from build123d import *

# Parameters (mm, degrees)
BOSS_EXTRUDE7_DEPTH = 40
BOSS_EXTRUDE8_DEPTH = 10
SKETCH16_R          = 4
CUT_EXTRUDE6_DEPTH  = 93.663838512
SKETCH17_R          = 4.375
CUT_EXTRUDE7_DEPTH  = 10
FILLET2_R           = 5
MIRROR2_START       = 14.3750001
MIRROR2_DEPTH       = 6.6249998
MIRROR2_2_DEPTH     = 10
MIRROR2_START_2     = 5
MIRROR2_3_DEPTH     = 0.6249999
MIRROR2_START_3     = 34.3750001
MIRROR2_4_DEPTH     = 0.6249999
MIRROR2_5_DEPTH     = 40
MIRROR2_START_4     = -9.5
MIRROR2_6_OUTLINE_R = 4.375
MIRROR2_6_DEPTH     = 8
MIRROR2_START_5     = 18.089296501
MIRROR2_7_OUTLINE_R = 4
MIRROR2_7_DEPTH     = 10.910703499


with BuildPart() as part:
    # Sketch15 → Boss-Extrude7 (new body)
    with BuildSketch(Plane(origin=(0, 0, 0), x_dir=(0, 0, -1), z_dir=(0, 1, 0))):
        with BuildLine():
            Line((33, 0), (39.3, 0))
            Line((39.3, 0), (69, -29.7))
            Line((69, -29.7), (55.282128445, -29.7))
            Line((55.282128445, -29.7), (40.368228689, -14.786100244))
            Line((40.368228689, -14.786100244), (27.577164466, -27.577164466))
            ThreePointArc((27.577164466, -27.577164466), (-10.389986255, -37.590533191), (-37.825256113, -9.5))
            Line((-37.825256113, -9.5), (-52.815891464, -9.5))
            Line((-52.815891464, -9.5), (-52.815891464, -1.5))
            Line((-52.815891464, -1.5), (-32.965891464, -1.5))
            ThreePointArc((-32.965891464, -1.5), (0.750193874, -32.991471764), (33, 0))
        make_face()
    extrude(amount=BOSS_EXTRUDE7_DEPTH)

    # Sketch15_4 → Boss-Extrude8 (add)
    with BuildSketch(Plane(origin=(0, 0, 0), x_dir=(0, 0, -1), z_dir=(0, 1, 0))):
        with BuildLine():
            ThreePointArc((27.577164466, -27.577164466), (26.44822372, -28.661672353), (25.276669084, -29.7))
            Line((25.276669084, -29.7), (55.282128445, -29.7))
            Line((55.282128445, -29.7), (40.368228689, -14.786100244))
            Line((40.368228689, -14.786100244), (27.577164466, -27.577164466))
        make_face()
    extrude(amount=BOSS_EXTRUDE8_DEPTH)

    # Sketch16 → Cut-Extrude6 (cut, through all)
    with BuildSketch(Plane(origin=(-12.791064222, 0, -12.791064222), x_dir=(-0.707106781186546, 0, 0.707106781186549), z_dir=(0.707106781186549, 0, 0.707106781186546))):
        with Locations(Location((-53.189296501, -25, 0), (0, 0, 180))):
            Circle(SKETCH16_R)
    extrude(amount=-CUT_EXTRUDE6_DEPTH, mode=Mode.SUBTRACT)

    # Sketch17 → Cut-Extrude7 (cut)
    with BuildSketch(Plane(origin=(0, 0, 0), x_dir=(0, -1, 0), z_dir=(1, 0, 0))):
        with Locations(Location((-30, -45.320573788, 0), (0, 0, 270))):
            Circle(SKETCH17_R)
        with Locations(Location((-10, -45.320573788, 0), (0, 0, 270))):
            Circle(SKETCH17_R)
    extrude(amount=CUT_EXTRUDE7_DEPTH, mode=Mode.SUBTRACT)

    # Fillet2
    fillet2_edges = [part.edges().sort_by_distance(p)[0] for p in [
        (5.5, 0, 52.815891464),
        (5.5, 40, 52.815891464),
        (14.786100244, 25, -40.368228689),
    ]]
    fillet(fillet2_edges, radius=FILLET2_R)

    # Mirror2: read off the stored shape, not the designer's step
    # Mirror2 outline → Mirror2 (add)
    with BuildSketch(Plane(origin=(0, 0, 0), x_dir=(1, 0, 0), z_dir=(0, 1, 0)).offset(MIRROR2_START)):
        with BuildLine():
            ThreePointArc((-27.577164466, 27.577164466), (-37.590533191, -10.389986255), (-9.5, -37.825256113))
            Line((-9.5, -37.825256113), (-9.5, -52.815891464))
            Line((-9.5, -52.815891464), (-1.5, -52.815891464))
            Line((-1.5, -52.815891464), (-1.5, -32.965891464))
            ThreePointArc((-1.5, -32.965891464), (-32.991471764, 0.750193874), (0, 33))
            Line((0, 33), (0, 39.3))
            Line((0, 39.3), (-29.7, 69))
            Line((-29.7, 69), (-29.7, 55.282128445))
            Line((-29.7, 55.282128445), (-18.32163415, 43.903762595))
            ThreePointArc((-18.32163415, 43.903762595), (-16.857168056, 40.368228689), (-18.32163415, 36.832694783))
            Line((-18.32163415, 36.832694783), (-27.577164466, 27.577164466))
        make_face()
    extrude(amount=MIRROR2_DEPTH)



with BuildPart() as body_2:
    # Mirror2 2 outline → Mirror2 2 (new body)
    with BuildSketch(Plane(origin=(0, 0, 0), x_dir=(1, 0, 0), z_dir=(0, 1, 0))):
        with BuildLine():
            Line((-29.7, 55.282128445), (-29.7, 25.276669084))
            ThreePointArc((-29.7, 25.276669084), (-28.661672353, 26.448223719), (-27.577164466, 27.577164466))
            Line((-27.577164466, 27.577164466), (-18.32163415, 36.832694783))
            ThreePointArc((-18.32163415, 36.832694783), (-16.857168056, 40.368228689), (-18.32163415, 43.903762595))
            Line((-18.32163415, 43.903762595), (-29.7, 55.282128445))
        make_face()
    extrude(amount=MIRROR2_2_DEPTH)


with BuildPart() as part_1:
    add(part.part)

    add(body_2.part)  # Mirror2 3 merges body 2
    # Mirror2 3 outline → Mirror2 3 (add)
    with BuildSketch(Plane(origin=(0, 0, 0), x_dir=(1, 0, 0), z_dir=(0, 1, 0)).offset(MIRROR2_START_2)):
        with BuildLine():
            ThreePointArc((-27.577164466, 27.577164466), (-37.590533191, -10.389986255), (-9.5, -37.825256113))
            Line((-9.5, -37.825256113), (-9.5, -52.815891464))
            Line((-9.5, -52.815891464), (-1.5, -52.815891464))
            Line((-1.5, -52.815891464), (-1.5, -32.965891464))
            ThreePointArc((-1.5, -32.965891464), (-32.991471764, 0.750193874), (0, 33))
            Line((0, 33), (0, 39.3))
            Line((0, 39.3), (-29.7, 69))
            Line((-29.7, 69), (-29.7, 55.282128445))
            Line((-29.7, 55.282128445), (-18.32163415, 43.903762595))
            ThreePointArc((-18.32163415, 43.903762595), (-16.857168056, 40.368228689), (-18.32163415, 36.832694783))
            Line((-18.32163415, 36.832694783), (-27.577164466, 27.577164466))
        make_face()
    extrude(amount=MIRROR2_3_DEPTH)

    # Mirror2 4 outline → Mirror2 4 (add)
    with BuildSketch(Plane(origin=(0, 0, 0), x_dir=(1, 0, 0), z_dir=(0, 1, 0)).offset(MIRROR2_START_3)):
        with BuildLine():
            ThreePointArc((-27.577164466, 27.577164466), (-37.590533191, -10.389986255), (-9.5, -37.825256113))
            Line((-9.5, -37.825256113), (-9.5, -52.815891464))
            Line((-9.5, -52.815891464), (-1.5, -52.815891464))
            Line((-1.5, -52.815891464), (-1.5, -32.965891464))
            ThreePointArc((-1.5, -32.965891464), (-32.991471764, 0.750193874), (0, 33))
            Line((0, 33), (0, 39.3))
            Line((0, 39.3), (-29.7, 69))
            Line((-29.7, 69), (-29.7, 55.282128445))
            Line((-29.7, 55.282128445), (-18.32163415, 43.903762595))
            ThreePointArc((-18.32163415, 43.903762595), (-16.857168056, 40.368228689), (-18.32163415, 36.832694783))
            Line((-18.32163415, 36.832694783), (-27.577164466, 27.577164466))
        make_face()
    extrude(amount=MIRROR2_4_DEPTH)

    # Mirror2 5 outline → Mirror2 5 (add)
    with BuildSketch(Plane(origin=(0, 0, 0), x_dir=(1, 0, 0), z_dir=(0, 1, 0))):
        with BuildLine():
            ThreePointArc((-27.577164465, 27.577164467), (-37.590533191, -10.389986254), (-9.5, -37.825256113))
            Line((-9.5, -37.825256113), (-9.5, -52.815891464))
            Line((-9.5, -52.815891464), (-1.5, -52.815891464))
            Line((-1.5, -52.815891464), (-1.5, -32.965891464))
            ThreePointArc((-1.5, -32.965891464), (-32.991471764, 0.750193874), (0, 33))
            Line((0, 33), (0, 39.3))
            Line((0, 39.3), (-29.7, 69))
            Line((-29.7, 69), (-29.7, 55.282128445))
            Line((-29.7, 55.282128445), (-18.32163415, 43.903762595))
            ThreePointArc((-18.32163415, 43.903762595), (-16.857168056, 40.368228689), (-18.32163415, 36.832694783))
            Line((-18.32163415, 36.832694783), (-27.577164465, 27.577164467))
        make_face()
    extrude(amount=MIRROR2_5_DEPTH)

    # Mirror2 6 outline → Mirror2 6 (cut)
    with BuildSketch(Plane.YZ.offset(MIRROR2_START_4)):
        with Locations((30, 45.320573788)):
            Circle(MIRROR2_6_OUTLINE_R)
        with Locations((10, 45.320573788)):
            Circle(MIRROR2_6_OUTLINE_R)
        with BuildLine():
            Line((0, 52.815891464), (0, 47.815891464))
            ThreePointArc((0, 47.815891464), (1.464466094, 51.35142537), (5, 52.815891464))
            Line((5, 52.815891464), (0, 52.815891464))
        make_face()
        with BuildLine():
            Line((40, 52.815891464), (35, 52.815891464))
            ThreePointArc((35, 52.815891464), (38.535533906, 51.35142537), (40, 47.815891464))
            Line((40, 47.815891464), (40, 52.815891464))
        make_face()
    extrude(amount=MIRROR2_6_DEPTH, mode=Mode.SUBTRACT)

    # Mirror2 7 outline → Mirror2 7 (cut)
    with BuildSketch(Plane(origin=(0, 0, 0), x_dir=(0.707106781186546, 0, 0.707106781186549), z_dir=(0.707106781186549, 0, -0.707106781186546)).offset(MIRROR2_START_5)):
        with Locations((-53.189296501, -25)):
            Circle(MIRROR2_7_OUTLINE_R)
    extrude(amount=MIRROR2_7_DEPTH, mode=Mode.SUBTRACT)


solid = part_1.part
Geometry: final body of the model. Coordinates: model frame, mm. A direction names the side the tool comes from. Give positions to 0.01 mm unless a question says otherwise; leave off trailing zeros. Write each loop counter-clockwise with the first axis right and the second up, starting at its lowest first coordinate (ties: lowest second). Pieces come first, ordered by that corner, then holes.
(1) Ray query, line 1 (Z direction, x = -6, y = 30); line 2 (Z direction, x = -27, y = 23); line 3 (X direction, y = 5, z = -9.5). Return the intervals inside material, ascending.
(2) Cut plane D-D, the plane z = 15. Return loops of the section in (x, y).
(3) Mould query, pull axis Z, two halves, no side actions, for faces 1 (the cylindrical face through (5.4, 28.7, 49.5)), 2 (the cylindrical face through (-5.556, 38.496, 51.39)), 3 (the flat face through (1.5, 20, 43)), 4 (the flat face through (-14.6, 19.7, -53.9)). Classes: released by +Z, released by -Z, zero draft, split by the parting line, or undercut.
(4) First-contact query: P1, Ø1.5, axis at x = -30, y = 9.5, coming from the -Z side; P2, Ø6, axis at y = 14, z = -14, coming from the +X side; P3, Ø1, axis at y = 14, z = -18, coming from the +X side; P4, Ø14, axis at x = 21, z = -44.5, coming from the +Y side. Flat tips, straight axial feed; report the tip coordinate or a pass-through.
(5) Cut plane A-A, the plane x = -3.5. Return loops of the section in (y, z) (3 decimals), then the cut area to 3 significant figures.
(6) Cut plane C-C, the plane y = 22.5. Return loops of the section in (x, z).
(7) Cut plane B-B, the plane z = 0. Return loops of the section in (x, y), then the cut area to 3 significant figures.
(8) Access query for faces 5 (the flat face through (-29.7, 15, -57)), 6 (the flat face through (-9.5, 20, 45)), 7 (the cylindrical face through (-16.857, 24.79, -40.423)), 8 (the cylindrical face through (16.857, 25.21, -40.423)), 9 (the flat face through (29.7, 15, -57)). Directions: +Z, -Z, +X, -X, +Y, -Y. A direction counts if a zero-diameter tool reaches every point of the face in a straight line with its end or side. Return the directions, or none.
Values follow:
1. line 1: z = -45.3 to -32.45, 32.45 to 40.95, 49.7 to 52.82
1. line 2: z = -66.3 to -53.12, -28.15 to -18.97, 18.97 to 28.14
1. line 3: x = -37.83 to -31.6, 31.6 to 37.83
2. outline: (-36, 0) - (-29.39, 0) - (-29.39, 40) - (-36, 40) - close; (29.39, 0) - (36, 0) - (36, 40) - (29.39, 40) - close
3. face 1: undercut
3. face 2: released by +Z
3. face 3: zero draft
3. face 4: released by -Z
4. P1: stops at z = -69
4. P2: stops at x = 37.42
4. P3: stops at x = 34.85
4. P4: stops at y = 40
5. outline: (0, -42.8) - (40, -42.8) - (40, -32.814) - (0, -32.814) - close; (0, 32.814) - (40, 32.814) - (40, 47.816) arc R5 ccw to (35, 52.816) - (5, 52.816) arc R5 ccw to (0, 47.816) - close; hole circle Ø8.75 at (10, 45.321); hole circle Ø8.75 at (30, 45.321)
5. area: 1,070 mm2
6. outline: (-29.7, -69) - (-20.17, -59.47) - (-27.03, -52.61) - (-29.7, -55.28) - close; (-27.58, -27.58) - (-18.32, -36.83) arc R5 cw to (-18.32, -43.9) - (-22.61, -48.19) - (-15.75, -55.05) - (0, -39.3) - (15.75, -55.05) - (22.61, -48.19) - (18.32, -43.9) arc R5 cw to (18.32, -36.83) - (27.58, -27.58) arc R39 ccw to (9.5, 37.83) - (9.5, 52.82) - (1.5, 52.82) - (1.5, 32.97) arc R33 cw (long way) to (-1.5, 32.97) - (-1.5, 52.82) - (-9.5, 52.82) - (-9.5, 37.83) arc R39 ccw to start; (20.17, -59.47) - (29.7, -69) - (29.7, -55.28) - (27.03, -52.61) - close
7. outline: (-39, 0) - (-33, 0) - (-33, 40) - (-39, 40) - close; (33, 0) - (39, 0) - (39, 40) - (33, 40) - close
7. area: 480 mm2
8. face 5: -Z, -X, +Y, -Y
8. face 6: +Z, -X, +Y, -Y
8. face 7: -X, +Y
8. face 8: +X, +Y
8. face 9: -Z, +X, +Y, -Y
